Part print with two shaded views. Sizes in mm from the minimum x, y, z corner. A direction names the side the tool comes from. Coordinates: 2 decimals unless noted, no trailing zeros. Write each loop counter-clockwise with the first axis right and the second up, starting at its lowest first coordinate (ties: lowest second). Pieces come first, ordered by that corner, then holes.
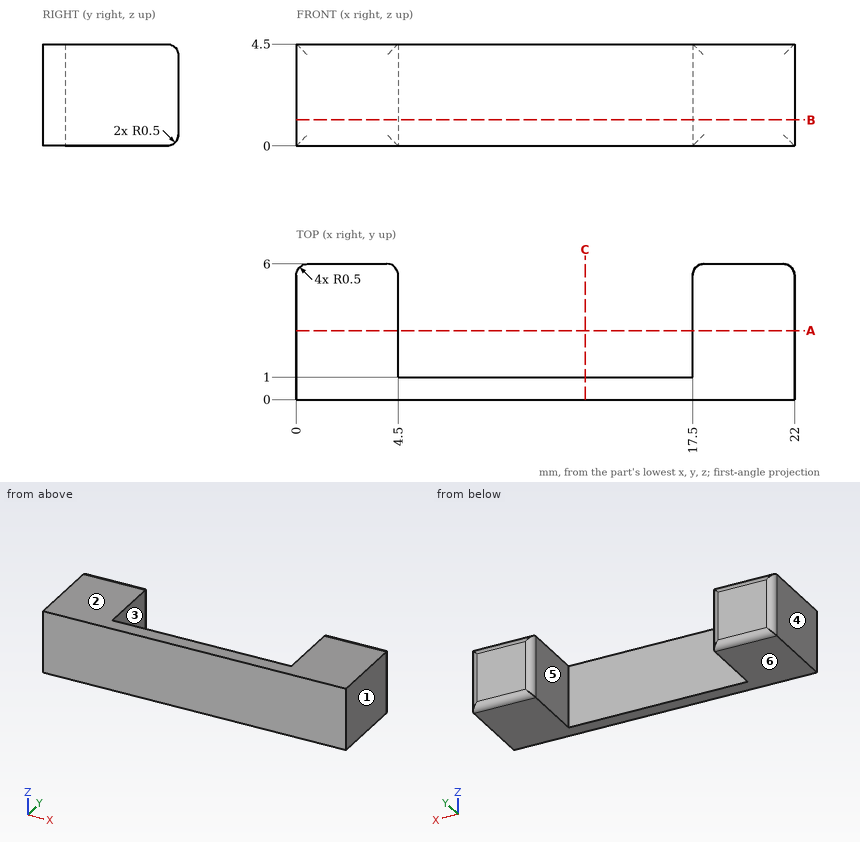
(1) Slice it at A-A, the plane y = 3.05. List the corners of the cut face in (x, z).
(2) Slice it at C-C, the plane x = 12.75. List the corners of the cut face in (y, z), and give its area (3 significant figures).
(3) Flat gauge pin, fed straight in: P1, Ø1, axis at x = 14, z = 1.5, coming from the +Y side. Where does the tip first touch, or does it go through?
(4) Slice it at B-B, the plane z = 1.15. List the corners of the cut face in (x, y).
(5) Probe L1, parallel to X at y = 2.7, z = 2.9; L2, parallel to Y at x = 10.75, z = 0.75; L3, parallel to Y at x = 4.25, z = 3.65. List the from-to ranges inside material, lowest first.
(6) Two-plate mould, pull along X, no slides. Class the marked faces 1, 2, 3 and 4: pulls with the +X half, pulls with the -X half, needs draft (parallel to the pull), parting line crosses it, or undercut.
(7) 3-axis set-ups, long thin cutter, end or side, ignore diameter. For the marked faces 5 and 6: which of +Z, -Z, +X, -X, +Y, -Y reach the whole face in a straight line?
Results:
1. outline: (0, 0) - (4.5, 0) - (4.5, 4.5) - (0, 4.5) - close; (17.5, 0) - (22, 0) - (22, 4.5) - (17.5, 4.5) - close
2. outline: (0, 0) - (1, 0) - (1, 4.5) - (0, 4.5) - close
2. area: 4.50 mm2
3. P1: stops at y = 1
4. outline: (0, 0) - (22, 0) - (22, 5.5) arc R0.5 ccw to (21.5, 6) - (18, 6) arc R0.5 ccw to (17.5, 5.5) - (17.5, 1) - (4.5, 1) - (4.5, 5.5) arc R0.5 ccw to (4, 6) - (0.5, 6) arc R0.5 ccw to (0, 5.5) - close
5. L1: x = 0 to 4.5, 17.5 to 22
5. L2: y = 0 to 1
5. L3: y = 0 to 5.93
6. face 1: pulls with the +X half
6. face 2: needs draft
6. face 3: undercut
6. face 4: pulls with the -X half
7. face 5: +Z, -Z, +Y
7. face 6: -Z, +X, -X, +Y, -Y
